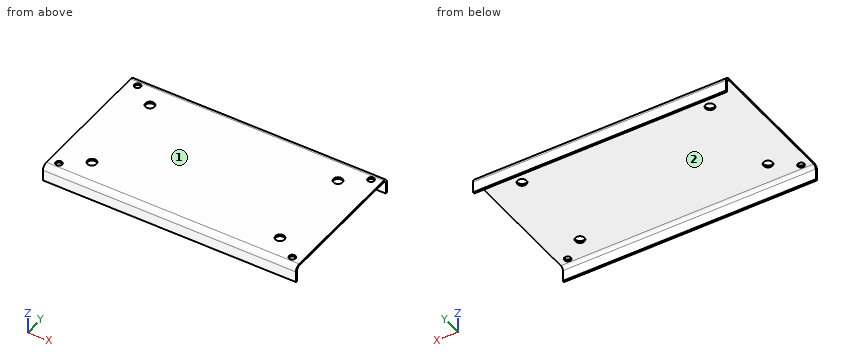
Autodesk Inventor part; units mm, degrees
ref_plane "YZ Plane" through (0, 0, 0) normal (1, 0, 0) x (0, 1, 0)
ref_plane "XZ Plane" through (0, 0, 0) normal (0, 1, 0) x (-1, 0, 0)
ref_plane "XY Plane" through (0, 0, 0) normal (0, 0, 1) x (1, 0, 0)
sketch "Sketch1" plane through (0, 0, 0) normal (0, 0, 1) x (1, 0, 0)
  line L0 (-195, 110) -> (195, 110)
  line L1 (195, 110) -> (195, -110)
  line L2 (195, -110) -> (-195, -110)
  line L3 (-195, -110) -> (-195, 110)
  line L4 (-195, 110) -> (195, -110) construction
  point P0 (0, 0)
  point P1 (0, 0)
  dimension "d0" = 390
  dimension "d1" = 220
extrude "Plate1" add sketch "Sketch1" against normal blind 3
sketch "Sketch2" plane through (0, 0, 0) normal (0, 0, 1) x (1, 0, 0)
  line L0 (-145, 70) -> (145, 70) construction
  line L1 (145, 70) -> (145, -70) construction
  line L2 (145, -70) -> (-145, -70) construction
  line L3 (-145, -70) -> (-145, 70) construction
  line L4 (195, -110) -> (195, 110)
  point P0 (0, 0)
  point P1 (-145, 0)
  point P2 (0, 70)
  dimension "d3" = 290
  dimension "d4" = 140
hole "Hole1" at (-145, 70, 0) at (145, 70, 0) at (-145, -70, 0) at (145, -70, 0) direction (0, 0, -1) diameter 14 end through all
sketch "Sketch3" plane through (0, 0, 0) normal (0, 0, 1) x (1, 0, 0)
  line L0 (-180, 95) -> (180, 95) construction
  line L1 (180, 95) -> (180, -95) construction
  line L2 (180, -95) -> (-180, -95) construction
  line L3 (-180, -95) -> (-180, 95) construction
  line L4 (-180, 95) -> (180, -95) construction
  point P0 (0, 0)
  point P1 (0, 0)
  dimension "d14" = 190
  dimension "d15" = 360
hole "Hole2" at (-180, 95, 0) at (180, 95, 0) at (180, -95, 0) at (-180, -95, 0) direction (0, 0, -1) diameter 10 end through all
sketch "Sketch4" plane through (-195, -107, 0) normal (0, -1, 0) x (1, 0, 0)
  line L0 (390, 0) -> (0, 0)
  line L1 (0, 0) -> (0, -25)
  line L2 (0, -25) -> (390, -25)
  line L3 (390, -25) -> (390, 0)
edge flange "Flange1" height 25 angle 90 thickness 3 bend radius 5 thickness toward (0, -1, 0) relief round relief width 3 relief depth 1.5 corner gap 5 corner form 0 edges at (0, -110, -3) (0, 110, -3) wall of the first edge with corners at (195, -107, 0) (-195, -107, 0) (-195, -107, -25) (195, -107, -25)
bend "Bend1"
corner "Corner1"
equation "\"d11\" = Thickness"
equation "\"d2\" = Thickness"
equation "\"d23\" = BendReliefWidth"
equation "\"d24\" = BendReliefDepth"
equation "\"d25\" = MinimumRemnant"
equation "\"d26\" = TransitionRadius"
equation "\"d29\" = BendRadius"
equation "\"d30\" = CornerReliefSize"
equation "\"d31\" = GapSize"
equation "\"d32\" = JacobiRadiusSize"
equation "\"BendReliefWidth\" = Thickness"
equation "\"BendReliefDepth\" = 0.5 * Thickness"
equation "\"CornerReliefSize\" = 4 * Thickness"
equation "\"MinimumRemnant\" = 2 * Thickness"
equation "\"TransitionRadius\" = BendRadius"
equation "\"JacobiRadiusSize\" = BendRadius"
equation "\"GapSize\" = Thickness"
properties part number "AIRPUMP plate" material "Stainless Steel"
Design review of the part built by this model. Coordinates are the model's own, in mm. Face numbers are marked on the shaded views. A direction names the side the tool comes from. Coordinates: 2 decimals unless noted, no trailing zeros. Order: outer loops, then holes, each group sorted by start corner. A loop starts at its lowest first (then second) coordinate and runs counter-clockwise, first axis right, second up.
1) For the marked faces 1 and 2, list the 3-axis set-ups (+Z, -Z, +X, -X, +Y, -Y) from which the entire face can be reached by the end or side of a thin tool; tool diameter is ignored.
2) Take a section at A-A, the plane y = -70. Give the boundary of the cut face in (x, z), and give its area (3 significant figures).
3) Wall thickness on line 1 along X through (y, z) = (-95, -0.95); line 2 along X through (y, z) = (70, -1.6); line 3 along Y through (x, z) = (-161, -9.25): over which ranges is each line inside the solid? List them lowest first.
4) Clearance check with flat-ended pins moving along their axes: pin 1 (18 mm diameter, centred on x = 145, y = -70, fed in from -Z); pin 2 (16 mm diameter, centred on x = 180, y = -95, fed in from -Z); pin 3 (8 mm diameter, centred on x = -180, y = 95, fed in from -Z). State where each tip first meets the part, or that it passes through.
5) Take a section at C-C, the plane x = -180. Give the boundary of the cut face in (y, z).
6) Take a section at B-B, the plane z = -18. Give the boundary of the cut face in (x, y), and give its area (3 significant figures).
7) Take a section at D-D, the plane x = 25. Give the boundary of the cut face in (y, z).
Returned:
1. face 1: +Z, +X, -X, +Y, -Y
1. face 2: -Z, +X, -X
2. outline: (-195, -3) - (-152, -3) - (-152, 0) - (-195, 0) - close; (-138, -3) - (138, -3) - (138, 0) - (-138, 0) - close; (152, -3) - (195, -3) - (195, 0) - (152, 0) - close
2. area: 1,090 mm2
3. line 1: x = -195 to -185, -175 to 175, 185 to 195
3. line 2: x = -195 to -152, -138 to 138, 152 to 195
3. line 3: y = -110 to -107, 107 to 110
4. pin 1: stops at z = -3
4. pin 2: stops at z = -3.1
4. pin 3: passes through
5. outline: (-110, -25) - (-107, -25) - (-107, -8) arc R5 cw to (-102, -3) - (-100, -3) - (-100, 0) - (-102, 0) arc R8 ccw to (-110, -8) - close; (-90, -3) - (90, -3) - (90, 0) - (-90, 0) - close; (100, -3) - (102, -3) arc R5 cw to (107, -8) - (107, -25) - (110, -25) - (110, -8) arc R8 ccw to (102, 0) - (100, 0) - close
6. outline: (-195, -110) - (195, -110) - (195, -107) - (-195, -107) - close; (-195, 107) - (195, 107) - (195, 110) - (-195, 110) - close
6. area: 2,340 mm2
7. outline: (-110, -25) - (-107, -25) - (-107, -8) arc R5 cw to (-102, -3) - (102, -3) arc R5 cw to (107, -8) - (107, -25) - (110, -25) - (110, -8) arc R8 ccw to (102, 0) - (-102, 0) arc R8 ccw to (-110, -8) - close
